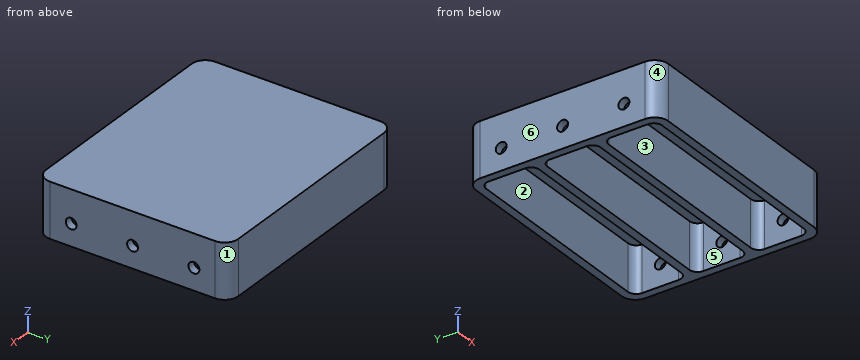
```python
from build123d import *

# Parameters (mm, degrees)
F0_W     = 86
F0_H     = 70.5
F0_W_2   = 80
F0_H_2   = 19.5
F1_DEPTH = 3
F2_DEPTH = 17
F4_D     = 4
F5_R     = 3
F6_R     = 5


with BuildPart() as f1:
    # F0 (on Top) → F1 (new body)
    with BuildSketch(Plane.XY):
        Rectangle(F0_W, F0_H)
        with Locations((0, -22.5)):
            Rectangle(F0_W_2, F0_H_2, mode=Mode.SUBTRACT)
        Rectangle(F0_W_2, F0_H_2, mode=Mode.SUBTRACT)
        with Locations((0, 22.5)):
            Rectangle(F0_W_2, F0_H_2, mode=Mode.SUBTRACT)
        with Locations((0, -22.5)):
            Rectangle(F0_W_2, F0_H_2)
        Rectangle(F0_W_2, F0_H_2)
        with Locations((0, 22.5)):
            Rectangle(F0_W_2, F0_H_2)
    extrude(amount=F1_DEPTH)

    # F0 (on Top) → F2 (join)
    with BuildSketch(Plane.XY):
        Rectangle(F0_W, F0_H)
        with Locations((0, -22.5)):
            Rectangle(F0_W_2, F0_H_2, mode=Mode.SUBTRACT)
        Rectangle(F0_W_2, F0_H_2, mode=Mode.SUBTRACT)
        with Locations((0, 22.5)):
            Rectangle(F0_W_2, F0_H_2, mode=Mode.SUBTRACT)
    extrude(amount=-F2_DEPTH)

    # F4 (through all)
    with Locations(Plane(origin=(-43, 0, 0), x_dir=(0, -1, 0), z_dir=(-1, 0, 0))):
        with Locations((-22.5, -9), (0, -9), (22.5, -9)):
            Hole(F4_D / 2)

    # F5
    f5_edges = [f1.edges().sort_by_distance(p)[0] for p in [
        (40, 32.25, -8.5),
        (-40, 32.25, -8.5),
        (-40, 12.75, -8.5),
        (40, 12.75, -8.5),
        (40, -9.75, -8.5),
        (-40, -9.75, -8.5),
        (-40, 9.75, -8.5),
        (40, 9.75, -8.5),
        (40, -12.75, -8.5),
        (-40, -12.75, -8.5),
        (-40, -32.25, -8.5),
        (40, -32.25, -8.5),
    ]]
    fillet(f5_edges, radius=F5_R)

    # F6
    f6_edges = [f1.edges().sort_by_distance(p)[0] for p in [
        (43, 35.25, -7),
        (43, -35.25, -7),
        (-43, -35.25, -7),
        (-43, 35.25, -7),
    ]]
    fillet(f6_edges, radius=F6_R)


solid = f1.part
```
Check sheet for the modelled part. Datum: model origin and axes. Units: mm. Face numbers are marked on the shaded views. A direction names the side the tool comes from. Coordinates: 2 decimals unless noted, no trailing zeros. Write each loop counter-clockwise with the first axis right and the second up, starting at its lowest first coordinate (ties: lowest second). Pieces come first, ordered by that corner, then holes. Notation, with made-up numbers: M 53.5,-6.75 L 80.5,-6.75 A19 ccw 80.5,-0.75 Z; hole C 76,51.25 d2. An arc over 180 degrees is marked long. Write item = value, one per line. Start each with the question number.
1. Sectioned sample at C-C (x = 27.5). Record the cut outline in (y, z), then the cut area to 4 significant figures.
2. Sectioned sample at A-A (z = -2.25). State how many separate pieces and enclosed holes the cut face has, then the cut area to 3 significant figures.
3. Sectioned sample at B-B (y = -22.5). Record the cut outline in (x, z), then the cut area to 3 significant figures.
4. Sectioned sample at D-D (y = -3.5). Record the cut outline in (x, z), then the cut area to 3 significant figures.
5. Mould release check, pull along X, two halves, no side actions. Record for the marked faces 1, 2, 3 and 4: pulls with the +X half, pulls with the -X half, needs draft (parallel to the pull), parting line crosses it, or undercut.
6. Thickness scan on probe 1 along Y at (x, z) = (13.5, -9.75); probe 2 along X at (y, z) = (16.5, -9.75); probe 3 along Z at (x, y) = (-41.05, 0). Record the ranges inside material, lowest first.
7. Go/stop test with a flat-tipped pin: pin 1 (1 mm diameter, centred on x = 23, y = -19.5, fed in from -Z). Record where the tip stops, or that it passes through.
8. Tool access check on the marked faces 5 and 6. Record the directions out of +Z, -Z, +X, -X, +Y, -Y that give a thin tool (end or side, any length) a straight path to the whole face; none if there is none.
The answers:
q1.outline = M -35.25,-17 L -32.25,-17 L -32.25,0 L -12.75,0 L -12.75,-17 L -9.75,-17 L -9.75,0 L 9.75,0 L 9.75,-17 L 12.75,-17 L 12.75,0 L 32.25,0 L 32.25,-17 L 35.25,-17 L 35.25,3 L -35.25,3 Z
q1.area = 415.5 mm²
q2.separate_pieces = 1
q2.enclosed_holes = 3
q2.area = 1,380 mm²
q3.outline = M -43,-17 L -40,-17 L -40,-11 L -43,-11 Z; M -43,-7 L -40,-7 L -40,0 L 40,0 L 40,-7 L 43,-7 L 43,3 L -43,3 Z; M 40,-17 L 43,-17 L 43,-11 L 40,-11 Z
q3.area = 336 mm²
q4.outline = M -43,-17 L -40,-17 L -40,0 L 40,0 L 40,-17 L 43,-17 L 43,3 L -43,3 Z
q4.area = 360 mm²
q5.face_1 = pulls with the +X half
q5.face_2 = undercut
q5.face_3 = undercut
q5.face_4 = pulls with the -X half
q6.probe_1 = -35.25 to -32.25, -12.75 to -9.75, 9.75 to 12.75, 32.25 to 35.25
q6.probe_2 = -43 to -40, 40 to 43
q6.probe_3 = -17 to -11, -7 to 3
q7.pin_1 = 0
q8.face_5 = -Z
q8.face_6 = +Z, -Z, -X, +Y, -Y
